Design review of the part built by this model. Coordinates are the model's own, in mm. A direction names the side the tool comes from. Coordinates: 2 decimals unless noted, no trailing zeros. Write each loop counter-clockwise with the first axis right and the second up, starting at its lowest first coordinate (ties: lowest second). Pieces come first, ordered by that corner, then holes. Notation, with made-up numbers: (-25, 73) -> (-15, 73) arc R24 cw to (-15, 87) -> close; hole circle Ø3 at (88, 15). An arc over 180 degrees is marked (long way). Answer in a Markdown table with one row per item. Add a question column.
Item 1: For faces 1 (the face through (0, -3, 8.6)), 2 (the face through (4.42, 1.54, 1.3)), list the 3-axis set-ups (+Z, -Z, +X, -X, +Y, -Y) from which the entire face can be reached by the end or side of a thin tool; tool diameter is ignored.
Item 2: Draft analysis for pull direction Y (two halves, no side actions). For faces 3 (the face through (0, 3, 0)), 4 (the face through (4.46, 0.59, 4.34)), 5 (the face through (-2.44, 0.54, 4.24)), state which applies: released by +Y, released by -Y, zero draft, split by the parting line, or undercut.
Item 3: To check wall thickness, follow line 1 (X direction, y = 0, z = 2.25); line 2 (Z direction, x = -5.5, y = 1.25); line 3 (X direction, y = 2.25, z = 8). State the ranges of each line that lie inside material, in increasing order.
Item 4: Clearance check with flat-ended pins moving along their axes: P1, Ø2, axis at x = -4, z = 6.5, coming from the -Y side; P2, Ø3, axis at y = -1.5, z = 6, coming from the +X side; P3, Ø5, axis at x = 2, z = 5.5, coming from the -Y side. State where each tip first meets the part, or that it passes through.
Item 5: Take a section at C-C, the plane x = 3.75. Write out the cut boundary in (y, z).
Item 6: Take a section at A-A, the plane x = 0. Write out the cut boundary in (y, z), and give its area (3 significant figures).
Item 7: Take a section at D-D, the plane z = 5.5. Write out the cut boundary in (x, y).
from build123d import *


with BuildPart() as part:
    # Sketch → Revolution (revolve)
    with BuildSketch(Plane.YZ):
        Polygon((-6.5, 8.6), (-2.5, 8.6), (-2.5, 0), (-6.5, 0), (-6.5, 1.3), (-4.5, 1.3), (-4.5, 7.3), (-6.5, 7.3), align=None)
    revolve(axis=Axis((0, 0, 0), (0, 0, 1)))


solid = part.part
Answers:
| question | item | result |
|---|---|---|
| 1 | face 1 | +Z, +X, -X, +Y, -Y |
| 1 | face 2 | none |
| 2 | face 3 | zero draft |
| 2 | face 4 | split by the parting line |
| 2 | face 5 | undercut |
| 3 | line 1 | x = -4.5 to -2.5, 2.5 to 4.5 |
| 3 | line 2 | z = 0 to 1.3, 7.3 to 8.6 |
| 3 | line 3 | x = -6.1 to -1.09, 1.09 to 6.1 |
| 4 | P1 | stops at y = -5.54 |
| 4 | P2 | stops at x = 6.46 |
| 4 | P3 | stops at y = -6.49 |
| 5 | outline | (-5.31, 0) -> (5.31, 0) -> (5.31, 1.3) -> (2.49, 1.3) -> (2.49, 7.3) -> (5.31, 7.3) -> (5.31, 8.6) -> (-5.31, 8.6) -> (-5.31, 7.3) -> (-2.49, 7.3) -> (-2.49, 1.3) -> (-5.31, 1.3) -> close |
| 6 | outline | (-6.5, 0) -> (-2.5, 0) -> (-2.5, 8.6) -> (-6.5, 8.6) -> (-6.5, 7.3) -> (-4.5, 7.3) -> (-4.5, 1.3) -> (-6.5, 1.3) -> close; (2.5, 0) -> (6.5, 0) -> (6.5, 1.3) -> (4.5, 1.3) -> (4.5, 7.3) -> (6.5, 7.3) -> (6.5, 8.6) -> (2.5, 8.6) -> close |
| 6 | area | 44.8 mm^2 |
| 7 | outline | circle Ø9 at (0, 0); hole circle Ø5 at (0, 0) |
